```python
from build123d import *

# Parameters (mm, degrees)
F0_W     = 397
F0_H     = 324
F1_DEPTH = 20
F2_W     = 380
F2_H     = 305
F3_DEPTH = 1
F4_W     = 235
F4_H     = 145
F5_DEPTH = 25


with BuildPart() as f1:
    # F0 (on Front) → F1 (new body)
    with BuildSketch(Plane.XZ):
        Rectangle(F0_W, F0_H)
    extrude(amount=F1_DEPTH)

    # F2 (on face) → F3 (cut)
    with BuildSketch(Plane.XZ.offset(20)):
        Rectangle(F2_W, F2_H)
    extrude(amount=-F3_DEPTH, mode=Mode.SUBTRACT)

    # F4 (on face) → F5 (join)
    with BuildSketch(Plane.XZ):
        with Locations((30, 4.5)):
            Rectangle(F4_W, F4_H)
    extrude(amount=-F5_DEPTH)


solid = f1.part
```
The model under review builds one solid part; all positions refer to its coordinate system, in mm. A direction names the side the tool comes from. Give positions to 0.01 mm unless a question says otherwise; leave off trailing zeros. Loops run counter-clockwise (first coordinate to the right, second up) from the corner with the lowest first, then second, coordinate; pieces in that order, holes last. Notation, with made-up numbers: (60.25, -1.5) -> (112.25, -1.5) arc R12 cw to (112.25, 17.5) -> close; hole circle Ø3 at (40.5, 25). An arc over 180 degrees is marked (long way). Use CSV: the item, a comma, the result in double quotes.
1. The part is to be moulded in two halves that separate along X. For faces 5 (the face through (-3, 0, -70)), 6 (the face through (-3, -19, 2)), 7 (the face through (-198.5, -10, -2)), say which applies: +X half, -X half, draft (parallel to the pull), parting line (faces both ways), or undercut.
Result:
face 5,"draft"
face 6,"undercut"
face 7,"-X half"
2. Machinability: for faces 1 (the face through (147.5, 12, 3)), 2 (the face through (28, 12, 77)), 3 (the face through (28, 12, -68)), 4 (the face through (-87.5, 12, 3)), which of the approach directions +Z, -Z, +X, -X, +Y, -Y give a long, thin tool a straight path to every point of the face, cutting with its end or side? Answer none if there is none.
Result:
face 1,"+Z, -Z, +X, +Y"
face 2,"+Z, +X, -X, +Y"
face 3,"-Z, +X, -X, +Y"
face 4,"+Z, -Z, -X, +Y"
3. Consider section A-A, the plane x = -130.5. Write out the cut boundary in (y, z).
Result:
outline,"(-20, -162) -> (0, -162) -> (0, 162) -> (-20, 162) -> (-20, 152.5) -> (-19, 152.5) -> (-19, -152.5) -> (-20, -152.5) -> close"
4. Consider section D-D, the plane z = -26. Write out the cut boundary in (x, y), then the cut area to 3 significant figures.
Result:
outline,"(-198.5, -20) -> (-190, -20) -> (-190, -19) -> (190, -19) -> (190, -20) -> (198.5, -20) -> (198.5, 0) -> (147.5, 0) -> (147.5, 25) -> (-87.5, 25) -> (-87.5, 0) -> (-198.5, 0) -> close"
area,"13,400 mm²"
5. Consider section C-C, the plane y = 6.5. Write out the cut boundary in (x, z).
Result:
outline,"(-87.5, -68) -> (147.5, -68) -> (147.5, 77) -> (-87.5, 77) -> close"
6. For P1, Ø12, axis at x = 25.5, z = -128, coming from the +Y side; P2, Ø20, axis at y = 17.5, z = 40.5, coming from the +X side; P3, Ø5, axis at y = 11, z = 44, coming from the -X side, all flat-tipped, find the tip position at first contact; note any pin that passes through.
Result:
P1,"stops at y = 0"
P2,"stops at x = 147.5"
P3,"stops at x = -87.5"
7. To check wall thickness, follow probe 1 along Y at (x, z) = (-118, -49); probe 2 along X at (y, z) = (19.5, 54); probe 3 along Z at (x, y) = (46, 15). State the ranges of each line that lie inside material, in increasing order. Write a range as from..to.
Result:
probe 1,"y = -19..0"
probe 2,"x = -87.5..147.5"
probe 3,"z = -68..77"
8. Consider section B-B, the plane z = 129. Write out the cut boundary in (x, y), then the cut area to 3 significant figures.
Result:
outline,"(-198.5, -20) -> (-190, -20) -> (-190, -19) -> (190, -19) -> (190, -20) -> (198.5, -20) -> (198.5, 0) -> (-198.5, 0) -> close"
area,"7,560 mm²"
